The model under review builds one solid part; all positions refer to its coordinate system, in mm. A direction names the side the tool comes from. Round coordinates to 2 decimals unless told otherwise and drop trailing zeros. Order: outer loops, then holes, each group sorted by start corner. A loop starts at its lowest first (then second) coordinate and runs counter-clockwise, first axis right, second up. Notation, with made-up numbers: M 70.25,38 L 87.25,38 A26 ccw 87.25,55 Z; hole C 10.25,-7.75 d1. An arc over 180 degrees is marked long. Answer as a JSON object with one key per item and string values. Group by question number.
1. Clearance check with flat-ended pins moving along their axes: P1, Ø1.2, axis at x = 500.5, y = 68.5, coming from the -Z side; P2, Ø8, axis at x = 342.5, y = 222.5, coming from the -Z side; P3, Ø3, axis at y = 52, z = 3, coming from the +X side; P4, Ø3, axis at y = 67.5, z = 12, coming from the -X side. State where each tip first meets the part, or that it passes through.
2. To check wall thickness, follow probe 1 along X at (y, z) = (21, 1.5); probe 2 along Z at (x, y) = (135.5, 225); probe 3 along Y at (x, z) = (32, 13.25). State the ranges of each line that lie inside material, in increasing order. Write a range as [from, to].
3. Machinability: for faces 1 (the face through (409.95, 180.82, 13.86)), 2 (the face through (499, 70, 14)), 3 (the face through (507.99, 68.03, 21.15)), which of the approach directions +Z, -Z, +X, -X, +Y, -Y give a long, thin tool a straight path to every point of the face, cutting with its end or side? Answer none if there is none.
4. Add section A-A on z = 9.25. State the section outline as (x, y) points.
5. Add section B-B on x = 316.5. State the section outline as (y, z) points.
```python
from build123d import *

# Parameters (mm, degrees)
BOSS_EXTRUDE1_DEPTH = 4
SKETCH7_W           = 336.995970405
SKETCH7_H           = 4
BOSS_EXTRUDE2_DEPTH = 20
BOSS_EXTRUDE3_DEPTH = 20
SKETCH9_W           = 4
SKETCH9_H           = 4
BOSS_EXTRUDE4_DEPTH = 20
SKETCH10_W          = 20
SKETCH10_H          = 4
BOSS_EXTRUDE5_DEPTH = 24
SKETCH12_W          = 20
SKETCH12_H          = 4
BOSS_EXTRUDE6_DEPTH = 24
FILLET1_R           = 10


with BuildPart() as part:
    # Sketch1 → Boss-Extrude1 (new body)
    with BuildSketch(Plane.XY):
        Polygon((0, 0), (0, 300), (337, 300), (487, 70), (487, 0), align=None)
    extrude(amount=BOSS_EXTRUDE1_DEPTH)

    # Sketch7 → Boss-Extrude2 (add)
    with BuildSketch(Plane.XY.offset(4)):
        with Locations((168.497985203, 298)):
            Rectangle(SKETCH7_W, SKETCH7_H)
    extrude(amount=BOSS_EXTRUDE2_DEPTH)

    # Sketch8 → Boss-Extrude3 (add)
    with BuildSketch(Plane.XY.offset(4)):
        Polygon((336.995970405, 300), (487, 70), (483.649584471, 67.814887695), (333.645554877, 297.814887695), align=None)
    extrude(amount=BOSS_EXTRUDE3_DEPTH)

    # Sketch9 → Boss-Extrude4 (add)
    with BuildSketch(Plane.XY.offset(4)):
        with Locations((485, 68)):
            Rectangle(SKETCH9_W, SKETCH9_H)
    extrude(amount=BOSS_EXTRUDE4_DEPTH)

    # Sketch10 → Boss-Extrude5 (add)
    with BuildSketch(Plane(origin=(487, 0, 0), x_dir=(0, 0, -1), z_dir=(1, 0, 0))):
        with Locations((-14, 68)):
            Rectangle(SKETCH10_W, SKETCH10_H)
    extrude(amount=BOSS_EXTRUDE5_DEPTH)

    # Sketch12 → Boss-Extrude6 (add)
    with BuildSketch(Plane.ZY):
        with Locations((14, 298)):
            Rectangle(SKETCH12_W, SKETCH12_H)
    extrude(amount=BOSS_EXTRUDE6_DEPTH)

    # Fillet1
    fillet1_edges = [part.edges().sort_by_distance(p)[0] for p in [
        (511, 68, 24),
        (-24, 298, 24),
    ]]
    fillet(fillet1_edges, radius=FILLET1_R)


solid = part.part
```
Recorded:
{
 "1": {"P1": "stops at z = 4", "P2": "stops at z = 0", "P3": "stops at x = 487", "P4": "stops at x = 482.88"},
 "2": {"probe 1": "x = [0, 487]", "probe 2": "z = [0, 4]", "probe 3": "y = [296, 300]"},
 "3": {"face 1": "+Z, -X, -Y", "face 2": "+Z, -Z, +X, +Y", "face 3": "+Z, +X, +Y, -Y"},
 "4": {"outline": "M -24,296 L 334.83,296 L 483,68.81 L 483,66 L 511,66 L 511,70 L 487,70 L 337,300 L -24,300 Z"},
 "5": {"outline": "M 0,0 L 300,0 L 300,24 L 296,24 L 296,4 L 0,4 Z"}
}
